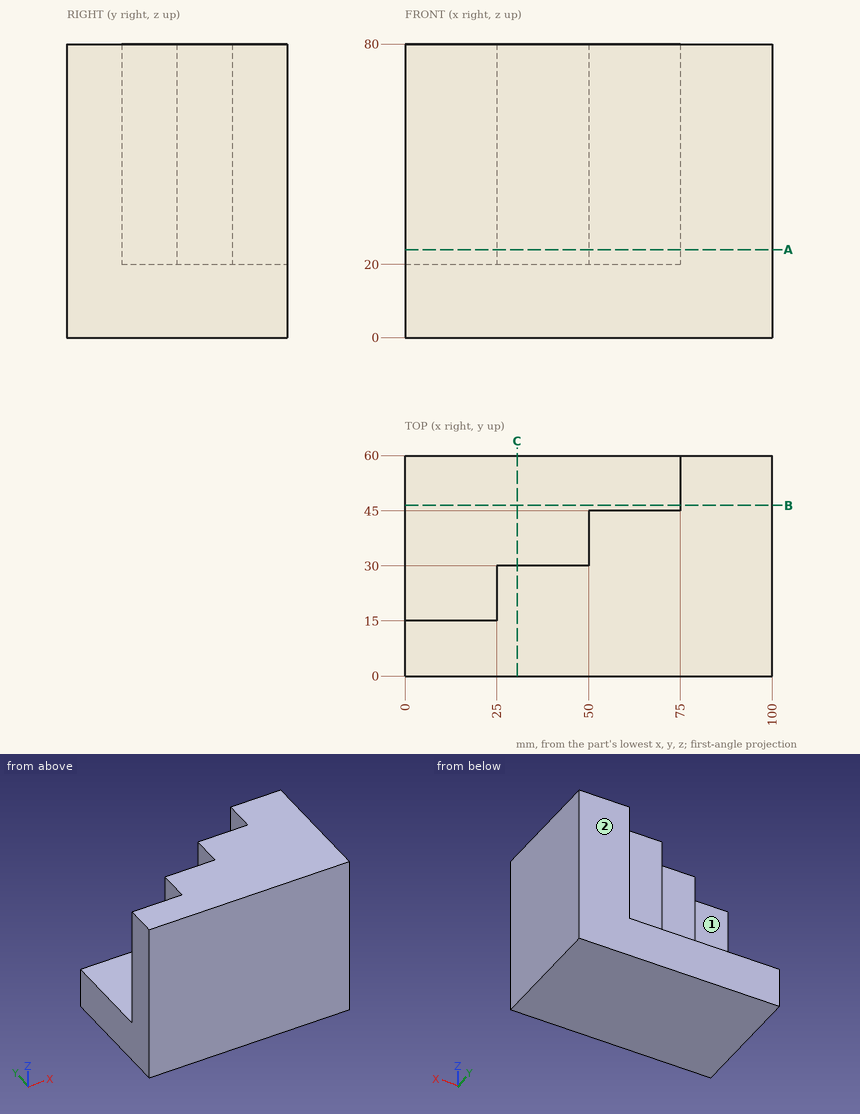
Verification items for this drawing (mm, ordinates from the low corner). A direction names the side the tool comes from. Coordinates: 2 decimals unless noted, no trailing zeros. Loops run counter-clockwise (first coordinate to the right, second up) from the corner with the lowest first, then second, coordinate; pieces in that order, holes last. Notation, with made-up numbers: (44.25, -23) - (80.25, -23) arc R24 cw to (80.25, 4) - close; hole circle Ø4 at (-32.75, 61.25). An arc over 180 degrees is marked (long way). Use one line per item in the form item = value. Start each with the question number.
Item 1: Section check B-B, the plane y = 46.5. Enter the section's corners in (x, z).
Item 2: Section check C-C, the plane x = 30.5. Enter the section's corners in (y, z), and give its area (3 significant figures).
Item 3: Gauge pin test, flat ends, axial feed: pin 1 (5 mm diameter, centred on y = 13.5, z = 22.5, fed in from -X); pin 2 (12.5 mm diameter, centred on x = 16, z = 61, fed in from +Y); pin 3 (16.5 mm diameter, centred on y = 24.5, z = 45, fed in from -X); pin 4 (1.5 mm diameter, centred on y = 43, z = 30, fed in from -X). Record the tip position at first contact, or that the pin passes through.
Item 4: Section check A-A, the plane z = 24. Enter the section's corners in (x, y), and give its area (3 significant figures).
Item 5: Tool access check on the marked faces 1 and 2. Record the directions out of +Z, -Z, +X, -X, +Y, -Y that give a thin tool (end or side, any length) a straight path to the whole face; none if there is none.
Item 6: Thickness scan on probe 1 along X at (y, z) = (26, 55); probe 2 along Y at (x, z) = (38, 36.5); probe 3 along Z at (x, y) = (25.5, 51). Record the ranges inside material, lowest first.
Computed:
q1.outline = (0, 0) - (100, 0) - (100, 80) - (75, 80) - (75, 20) - (0, 20) - close
q2.outline = (0, 0) - (60, 0) - (60, 20) - (30, 20) - (30, 80) - (0, 80) - close
q2.area = 3,000 mm2
q3.pin_1 = 0
q3.pin_2 = 15
q3.pin_3 = 25
q3.pin_4 = 50
q4.outline = (0, 0) - (100, 0) - (100, 60) - (75, 60) - (75, 45) - (50, 45) - (50, 30) - (25, 30) - (25, 15) - (0, 15) - close
q4.area = 3,750 mm2
q5.face_1 = +Z, -X, +Y
q5.face_2 = +Z, -Z, +X, -X, +Y
q6.probe_1 = 25 to 100
q6.probe_2 = 0 to 30
q6.probe_3 = 0 to 20
